The listing builds one solid part. Answer for the finished solid, in the listing's coordinates (mm). A direction names the side the tool comes from. Coordinates: 2 decimals unless noted, no trailing zeros. Write each loop counter-clockwise with the first axis right and the second up, starting at its lowest first coordinate (ties: lowest second). Pieces come first, ordered by that corner, then holes. Notation, with made-up numbers: M 27.5,-18 L 86.5,-18 A19 cw 86.5,19 Z; hole C 54,-3.5 d4. An arc over 180 degrees is marked long. Answer as CSV lines item,"result".
```python
from build123d import *

# Parameters (mm, degrees)
F1_DEPTH  = 152.4
F2_R      = 3.175
F3_DEPTH  = 152.401
F5_DEPTH  = 152.401
F6_R      = 2.54
F7_DEPTH  = 152.401
F8_DEPTH  = 152.4
F9_W      = 152.4
F9_H      = 101.6
F10_DEPTH = 82.3067692308


# Not quite as in the source:
# - a feature names something its author has since deleted; it is built from what else it names


with BuildPart() as f1:
    # F0 (on Front) → F1 (new body)
    with BuildSketch(Plane.XZ):
        with BuildLine():
            ThreePointArc((-2.11e-07, -88.9), (62.8617927729, -62.8617929221), (88.9, 0))
            ThreePointArc((88.9, 0), (62.8617928475, 62.8617928475), (0, 88.9))
            ThreePointArc((0, 88.9), (-62.8617927742, 62.8617929208), (-88.9, 2.073e-07))
            ThreePointArc((-88.9, 2.073e-07), (-62.8617929954, -62.8617926996), (-2.11e-07, -88.9))
        make_face()
    extrude(amount=-F1_DEPTH)

    # F2 (on face) → F3 (cut, through all)
    with BuildSketch(Plane.XZ):
        with Locations((0, -82.55)):
            Circle(F2_R)
        with Locations((82.55, 0)):
            Circle(F2_R)
        with Locations((-82.55, 0)):
            Circle(F2_R)
    extrude(amount=-F3_DEPTH, mode=Mode.SUBTRACT)

    # F4 (on face) → F5 (cut, through all)
    with BuildSketch(Plane.XZ):
        Polygon((-94.202041626, 6.35), (0, 6.35), (132.5988769531, 6.35), (114.2803505063, 107.1024313569), (-94.202041626, 107.1024313569), align=None)
    extrude(amount=-F5_DEPTH, mode=Mode.SUBTRACT)

    # F6 (on face) + F2 (on face) → F7 (cut, through all)
    with BuildSketch(Plane.XZ):
        with Locations((-85.598, 6.35)):
            Circle(F6_R)
        with BuildLine():
            ThreePointArc((88.138, 6.35), (85.598, 8.89), (83.058, 6.35))
            ThreePointArc((83.058, 6.35), (85.598, 3.81), (88.138, 6.35))
        make_face()
    with BuildSketch(Plane.XZ):
        with BuildLine():
            Line((0, 43.9940905122), (-76.2, 0))
            ThreePointArc((-76.2, 0), (-77.974338005, -4.4029328075), (-82.3057692308, -6.3453015162))
            ThreePointArc((-82.3057692308, -6.3453015162), (-58.3716647869, -58.3716647869), (-6.3453015162, -82.3057692308))
            ThreePointArc((-6.3453015162, -82.3057692308), (0, -76.2), (6.3453015162, -82.3057692308))
            ThreePointArc((6.3453015162, -82.3057692308), (58.3716647869, -58.3716647869), (82.3057692308, -6.3453015162))
            ThreePointArc((82.3057692308, -6.3453015162), (77.974338005, -4.4029328075), (76.2, 0))
            Line((76.2, 0), (0, 43.9940905122))
        make_face()
    extrude(amount=-F7_DEPTH, mode=Mode.SUBTRACT)

    # F2 (on face) → F8 (join)
    with BuildSketch(Plane.XZ):
        with BuildLine():
            Line((0, 53.8645595374), (-25.4, 53.8645595374))
            Line((-25.4, 53.8645595374), (-25.4, 39.1998627))
            Line((-25.4, 39.1998627), (-82.3057692308, 6.3453015162))
            ThreePointArc((-82.3057692308, 6.3453015162), (-77.974338005, 4.4029328075), (-76.2, 0))
            Line((-76.2, 0), (0, 43.9940905122))
            Line((0, 43.9940905122), (76.2, 0))
            ThreePointArc((76.2, 0), (77.974338005, 4.4029328075), (82.3057692308, 6.3453015162))
            Line((82.3057692308, 6.3453015162), (25.4, 39.1998627))
            Line((25.4, 39.1998627), (25.4, 53.8645595374))
            Line((25.4, 53.8645595374), (0, 53.8645595374))
        make_face()
        with BuildLine():
            ThreePointArc((6.3453015162, 82.3057692308), (0, 76.2), (-6.3453015162, 82.3057692308))
            Line((-6.3453015162, 82.3057692308), (-25.4, 53.8645595374))
            Line((-25.4, 53.8645595374), (0, 53.8645595374))
            Line((0, 53.8645595374), (25.4, 53.8645595374))
            Line((25.4, 53.8645595374), (6.3453015162, 82.3057692308))
        make_face()
    extrude(amount=-F8_DEPTH)

    # F9 (on Top) → F10 (cut, through all)
    with BuildSketch(Plane.XY):
        with Locations((0, 76.2)):
            Rectangle(F9_W, F9_H)
    extrude(amount=F10_DEPTH, mode=Mode.SUBTRACT)


solid = f1.part
```
Q1. Find section A-A (z = 29). Give the vertices of the cut face in (x, y).
Output:
outline,"M -43.07,0 L -25.97,0 L -25.97,25.4 L -43.07,25.4 Z; M -43.07,127 L -25.97,127 L -25.97,152.4 L -43.07,152.4 Z; M 25.97,0 L 43.07,0 L 43.07,25.4 L 25.97,25.4 Z; M 25.97,127 L 43.07,127 L 43.07,152.4 L 25.97,152.4 Z"
Q2. Straight lines are drawn through the part: line 1 (Y direction, x = -4, z = 61); line 2 (Z direction, x = 0, y = 36) (3 decimals); line 3 (X direction, y = 19, z = -20.5). For each, find the intervals that lie inside material, in ascending order.
Output:
line 1,"0 to 25.4, 127 to 152.4"
line 2,"-88.9 to -85.725, -79.375 to -76.2"
line 3,"-86.5 to -79.96, 79.96 to 86.5"
Q3. For faces 1 (the cylindrical face through (0.1, 12.5, 76.2)), 2 (the flat face through (76.2, 75, 5)), 3 (the cylindrical face through (57.79, 75.13, -58.95)), 4 (the flat face through (25.4, 13, 46)), 5 (the flat face through (-25.4, 13, 47)), determine the directions among +Z, -Z, +X, -X, +Y, -Y from which every point of the face is accessible in a straight line to the end or side of a thin tool.
Output:
face 1,"+Z, +Y, -Y"
face 2,"+Z"
face 3,"+Y, -Y"
face 4,"+Z, +X, +Y, -Y"
face 5,"+Z, -X, +Y, -Y"
Q4. The mould has two halves that part along Z. Classify faces 6 (the cylindrical face through (-0.1, 75.1, -76.2)), 7 (the flat face through (-78.738, 58.2, 8.405)), 8 (the flat face through (-25.4, 140, 47)): pulls with the +Z half, pulls with the -Z half, needs draft (parallel to the pull), parting line crosses it, or undercut.
Output:
face 6,"undercut"
face 7,"pulls with the +Z half"
face 8,"needs draft"
Q5. Find section B-B (x = -51). Give the vertices of the cut face in (y, z), and give its area (3 significant figures).
Output:
outline,"M 0,-72.82 L 152.4,-72.82 L 152.4,-64.91 L 0,-64.91 Z; M 0,14.55 L 25.4,14.55 L 25.4,24.42 L 0,24.42 Z; M 127,14.55 L 152.4,14.55 L 152.4,24.42 L 127,24.42 Z"
area,"1,710 mm2"
Q6. Flat-ended cylindrical pins translate along their axes: pin 1 Ø16 at (y, z) = (9, 44) entering from +X; pin 2 Ø1.5 at (y, z) = (59.5, 7.5) entering from +X; pin 3 Ø3 at (y, z) = (98.5, 5) entering from +X. Find the tip coordinate at first contact, or state that the pin passes through.
Output:
pin 1,"x = 30.94"
pin 2,"x = 81.6"
pin 3,"x = 88.83"
Q7. Find section C-C (y = 30.5). Give the vertices of the cut face in (x, z) (3 decimals), and give its area (3 significant figures).
Output:
outline,"M -88.673,6.35 A88.9 ccw long 88.673,6.35 L 88.138,6.35 A2.54 cw 83.058,6.35 L 82.298,6.35 L 76.2,9.87 L 76.2,0 A6.35 ccw 82.306,-6.345 A82.55 cw 6.345,-82.306 A6.35 ccw -6.345,-82.306 A82.55 cw -82.306,-6.345 A6.35 ccw -76.2,0 L -76.2,9.87 L -82.298,6.35 L -83.058,6.35 A2.54 cw -88.138,6.35 Z; hole C -82.55,0 d6.35; hole C 0,-82.55 d6.35; hole C 82.55,0 d6.35"
area,"1,900 mm2"
Q8. Find section D-D (z = 61). Give the vertices of the cut face in (x, y), and give its area (3 significant figures).
Output:
outline,"M -20.62,0 L 20.62,0 L 20.62,25.4 L -20.62,25.4 Z; M -20.62,127 L 20.62,127 L 20.62,152.4 L -20.62,152.4 Z"
area,"2,090 mm2"
